Model file for the job. Use its own axes, mm. A direction names the side the tool comes from. Give positions to 0.01 mm unless a question says otherwise; leave off trailing zeros. Write each loop counter-clockwise with the first axis right and the second up, starting at its lowest first coordinate (ties: lowest second). Pieces come first, ordered by that corner, then holes. Notation, with made-up numbers: (-36, -24) - (0, -24) arc R19 cw to (0, -16) - close; hole circle Ø10 at (-28.5, 39.5). An arc over 180 degrees is marked (long way). One line per item, written item: value. Start each with the question number.
(1) Probe L1, parallel to Z at x = 0, y = 0.5; L2, parallel to Z at x = -1.5, y = 0.75; L3, parallel to Z at x = 2.5, y = 1.75. List the from-to ranges inside material, lowest first.
(2) Drop flat-ended pins along their axis: P1, Ø3, axis at x = 2, z = 12, coming from the -Y side; P2, Ø2, axis at x = 0.5, z = 3, coming from the -Y side; P3, Ø1, axis at y = 1.5, z = 1.5, coming from the -X side. Give the stop position or say it passes through.
(3) 3-axis set-ups, long thin cutter, end or side, ignore diameter. For faces 1 (the face through (0, 0, -1)), 2 (the face through (3, 1, 11)): which of +Z, -Z, +X, -X, +Y, -Y reach the whole face in a straight line?
(4) Mould opens along X. For faces 3 (the face through (0, 0, 21)), 4 (the face through (-2, 0, 15.5)), 5 (the face through (2.86, 0.9, 17.18)) say: pulls with the +X half, pulls with the -X half, needs draft (parallel to the pull), parting line crosses it, or undercut.
(5) Cut at D-D, the plane z = 2.75. List the corners of the cut face in (x, y).
(6) Cut at C-C, the plane y = 0. List the corners of the cut face in (x, z), and give its area (3 significant figures).
(7) Cut at B-B, the plane y = -2.75. List the corners of the cut face in (x, z), and give its area (3 significant figures).
(8) Cut at A-A, the plane x = 0. List the corners of the cut face in (y, z).
from build123d import *

# Parameters (mm, degrees)
CROQUIS1_R              = 3.5
SALIENTE_EXTRUIR1_DEPTH = 21
CROQUIS2_R              = 3.5
CROQUIS2_R_2            = 3
CORTAR_EXTRUIR1_DEPTH   = 10
CROQUIS3_R              = 2.5
CORTAR_EXTRUIR2_DEPTH   = 10
CROQUIS4_R              = 3.5
SALIENTE_EXTRUIR2_DEPTH = 1


with BuildPart() as part:
    # Croquis1 → Saliente-Extruir1 (new body)
    with BuildSketch(Plane.XY):
        Circle(CROQUIS1_R)
    extrude(amount=SALIENTE_EXTRUIR1_DEPTH)

    # Croquis2 → Cortar-Extruir1 (cut)
    with BuildSketch(Plane.XY.offset(21)):
        Circle(CROQUIS2_R)
        Circle(CROQUIS2_R_2, mode=Mode.SUBTRACT)
    extrude(amount=-CORTAR_EXTRUIR1_DEPTH, mode=Mode.SUBTRACT)

    # Croquis3 → Cortar-Extruir2 (cut)
    with BuildSketch(Plane(origin=(0, 0, 0), x_dir=(1, 0, 0), z_dir=(0, 1, 0))):
        with Locations((0, -14)):
            Circle(CROQUIS3_R)
    cortar_extruir2 = extrude(amount=-CORTAR_EXTRUIR2_DEPTH, mode=Mode.SUBTRACT)

    # Simetría1: Cortar-Extruir2 across plane
    add(cortar_extruir2.mirror(Plane.ZX), mode=Mode.SUBTRACT)

    # Croquis4 → Saliente-Extruir2 (add)
    with BuildSketch(Plane(origin=(0, 0, 0), x_dir=(-1, 0, 0), z_dir=(0, 0, -1))):
        Circle(CROQUIS4_R)
    extrude(amount=SALIENTE_EXTRUIR2_DEPTH)


solid = part.part
Answers follow:
1. L1: z = -1 to 11.5, 16.5 to 21
1. L2: z = -1 to 12, 16 to 21
1. L3: z = -1 to 11
2. P1: stops at y = -3.39
2. P2: stops at y = -3.5
2. P3: stops at x = -3.35
3. face 1: -Z, +X, -X, +Y, -Y
3. face 2: +Z
4. face 3: needs draft
4. face 4: undercut
4. face 5: parting line crosses it
5. outline: circle Ø7 at (0, 0)
6. outline: (-3.5, -1) - (3.5, -1) - (3.5, 11) - (3, 11) - (3, 21) - (-3, 21) - (-3, 11) - (-3.5, 11) - close; hole circle Ø5 at (0, 14)
6. area: 124 mm²
7. outline: (-2.17, -1) - (2.17, -1) - (2.17, 11) - (1.2, 11) - (1.2, 11.81) arc R2.5 cw to (-1.2, 11.81) - (-1.2, 11) - (-2.17, 11) - close; (-1.2, 16.19) arc R2.5 cw to (1.2, 16.19) - (1.2, 21) - (-1.2, 21) - close
7. area: 64.4 mm²
8. outline: (-3.5, -1) - (3.5, -1) - (3.5, 11) - (3, 11) - (3, 11.5) - (-3, 11.5) - (-3, 11) - (-3.5, 11) - close; (-3, 16.5) - (3, 16.5) - (3, 21) - (-3, 21) - close
